Source: three-view drawing plus pictorial views. Frame: mm from the lowest corner of the part. A direction names the side the tool comes from. Round coordinates to 2 decimals unless told otherwise and drop trailing zeros. Order: outer loops, then holes, each group sorted by start corner. A loop starts at its lowest first (then second) coordinate and runs counter-clockwise, first axis right, second up. Notation, with made-up numbers: (33, 88.25) -> (68, 88.25) arc R11 cw to (68, 92.25) -> close; hole circle Ø11 at (65.25, 72.5). An arc over 180 degrees is marked (long way). Use a Markdown table: item, result.
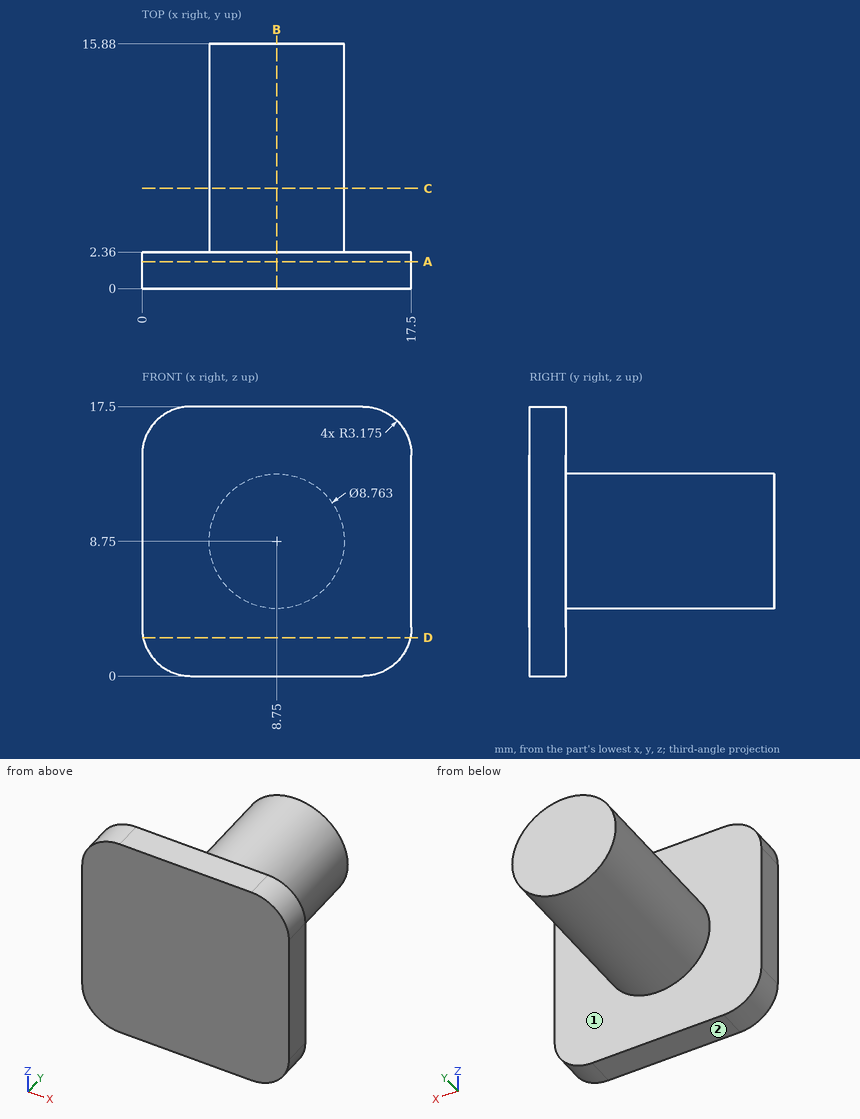
1) Cut plane D-D on z = 2.5. Return loops of the section in (x, y).
Results found:
| item | result |
|---|---|
| outline | (0.07, 0) -> (17.43, 0) -> (17.43, 2.36) -> (0.07, 2.36) -> close |
2) Pin query (flat end, axial travel): pin 1 Ø5 at (y, z) = (5.5, 15) entering from -X; pin 2 Ø1.5 at (y, z) = (13.5, 12) entering from +X; pin 3 Ø2 at (y, z) = (10, 6.5) entering from +X. Return the tip coordinate at first contact, or that it passes through.
Results found:
| item | result |
|---|---|
| pin 1 | stops at x = 6.48 |
| pin 2 | stops at x = 12.35 |
| pin 3 | stops at x = 12.95 |
3) Cut plane A-A on y = 1.75. Return loops of the section in (x, z) (3 decimals).
Results found:
| item | result |
|---|---|
| outline | (0, 3.175) arc R3.175 ccw to (3.175, 0) -> (14.325, 0) arc R3.175 ccw to (17.5, 3.175) -> (17.5, 14.325) arc R3.175 ccw to (14.325, 17.5) -> (3.175, 17.5) arc R3.175 ccw to (0, 14.325) -> close |
4) Cut plane C-C on y = 6.5. Return loops of the section in (x, z).
Results found:
| item | result |
|---|---|
| outline | circle Ø8.76 at (8.75, 8.75) |
5) Set-up query: the marked faces 1 and 2. Return all of +Z, -Z, +X, -X, +Y, -Y with unobstructed straight access to the full face (end or side cutting, diameter ignored); none if empty.
Results found:
| item | result |
|---|---|
| face 1 | +Y |
| face 2 | -Z, +X, -X, +Y, -Y |
6) Line query: L1, parallel to Y at x = 16.5, z = 6.5; L2, parallel to X at y = 9, z = 11.5; L3, parallel to X at y = 3.25, z = 9.5. Output: solid intervals per line, ascending. Write a range as [from, to].
Results found:
| item | result |
|---|---|
| L1 | y = [0, 2.36] |
| L2 | x = [5.34, 12.16] |
| L3 | x = [4.43, 13.07] |
7) Cut plane B-B on x = 8.75. Return loops of the section in (y, z).
Results found:
| item | result |
|---|---|
| outline | (0, 0) -> (2.36, 0) -> (2.36, 4.37) -> (15.88, 4.37) -> (15.88, 13.13) -> (2.36, 13.13) -> (2.36, 17.5) -> (0, 17.5) -> close |
